from build123d import *

# Parameters (mm, degrees)
SKETCH1_W           = 140.208
SKETCH1_H           = 150
BOSS_EXTRUDE1_DEPTH = 85.725
SKETCH2_W           = 30.48
SKETCH2_H           = 23.9522
SKETCH2_W_2         = 24.384
SKETCH2_H_2         = 17.8562
BOSS_EXTRUDE2_DEPTH = 3.048
SKETCH3_W           = 14.732
SKETCH3_H           = 20.828
BOSS_EXTRUDE3_DEPTH = 5.08
SKETCH4_R           = 1.27
CUT_EXTRUDE1_DEPTH  = 3.81
BOSS_EXTRUDE4_DEPTH = 3.048
SKETCH6_R           = 10.795
BOSS_EXTRUDE5_DEPTH = 25.4
SKETCH7_W           = 24.384
SKETCH7_H           = 17.8562
BOSS_EXTRUDE6_DEPTH = 43.18
SKETCH8_W           = 15.24
SKETCH8_H           = 11.43
BOSS_EXTRUDE7_DEPTH = 17.78
BOSS_EXTRUDE7_TAPER = 5


with BuildPart() as part:
    # Sketch1 → Boss-Extrude1 (new body)
    with BuildSketch(Plane(origin=(0, 0, 0), x_dir=(1, 0, 0), z_dir=(0, 1, 0))):
        with Locations((-120.400582929, 25.928824242)):
            Rectangle(SKETCH1_W, SKETCH1_H)
    extrude(amount=BOSS_EXTRUDE1_DEPTH)

    # Sketch2 → Boss-Extrude2 (add)
    with BuildSketch(Plane(origin=(-50.296582929, 0, 0), x_dir=(0, 0, -1), z_dir=(1, 0, 0))):
        with Locations((-28.243175758, 42.9641)):
            Rectangle(SKETCH2_W, SKETCH2_H)
        with Locations((-28.243175758, 42.9641)):
            Rectangle(SKETCH2_W_2, SKETCH2_H_2, mode=Mode.SUBTRACT)
    extrude(amount=BOSS_EXTRUDE2_DEPTH)

    # Sketch3 → Boss-Extrude3 (add)
    with BuildSketch(Plane(origin=(-50.296582929, 0, 0), x_dir=(0, 0, -1), z_dir=(1, 0, 0))):
        with Locations((-3.097175758, 43.0022)):
            Rectangle(SKETCH3_W, SKETCH3_H)
    extrude(amount=BOSS_EXTRUDE3_DEPTH)

    # Sketch4 → Cut-Extrude1 (cut)
    with BuildSketch(Plane(origin=(-50.296582929, 0, 0), x_dir=(0, 0, -1), z_dir=(1, 0, 0))):
        with Locations((-43.071175758, 6.35)):
            Circle(SKETCH4_R)
        with Locations((94.928824242, 6.35)):
            Circle(SKETCH4_R)
        with Locations((94.928824242, 70.35)):
            Circle(SKETCH4_R)
        with Locations((-19.071175758, 79.725)):
            Circle(SKETCH4_R)
    extrude(amount=-CUT_EXTRUDE1_DEPTH, mode=Mode.SUBTRACT)

    # Sketch5 → Boss-Extrude4 (add)
    with BuildSketch(Plane.ZY.offset(190.504582929)):
        with BuildLine():
            Line((49.071175758, 17.78), (26.211175758, 17.78))
            ThreePointArc((26.211175758, 17.78), (12.622175758, 31.369), (26.211175758, 44.958))
            Line((26.211175758, 44.958), (49.071175758, 44.958))
            Line((49.071175758, 44.958), (49.071175758, 17.78))
        make_face()
    extrude(amount=BOSS_EXTRUDE4_DEPTH)

    # Sketch6 → Boss-Extrude5 (add)
    with BuildSketch(Plane.ZY.offset(193.552582929)):
        with Locations((36.622716845, 31.369)):
            Circle(SKETCH6_R)
    extrude(amount=BOSS_EXTRUDE5_DEPTH)

    # Sketch7 → Boss-Extrude6 (add)
    with BuildSketch(Plane(origin=(-50.296582929, 0, 0), x_dir=(0, 0, -1), z_dir=(1, 0, 0))):
        with Locations((-28.243175758, 42.9641)):
            Rectangle(SKETCH7_W, SKETCH7_H)
    extrude(amount=BOSS_EXTRUDE6_DEPTH)

    # Sketch8 → Boss-Extrude7 (add)
    with BuildSketch(Plane(origin=(-7.116582929, 0, 0), x_dir=(0, 0, -1), z_dir=(1, 0, 0))):
        with Locations((-28.243175758, 42.9641)):
            Rectangle(SKETCH8_W, SKETCH8_H)
    extrude(amount=BOSS_EXTRUDE7_DEPTH, taper=BOSS_EXTRUDE7_TAPER)


solid = part.part
Verification items for the finished model (mm, model axes). A direction names the side the tool comes from. Round coordinates to 2 decimals unless told otherwise and drop trailing zeros. Write each loop counter-clockwise with the first axis right and the second up, starting at its lowest first coordinate (ties: lowest second). Pieces come first, ordered by that corner, then holes.
(1) Section check A-A (z = -43). Enter the section's corners in (x, y) (3 decimals).
Returned:
outline: (-190.505, 0) - (-50.297, 0) - (-50.297, 85.725) - (-190.505, 85.725) - close
(2) Depth check by flat-ended pin: pin 1 Ø3.5 at (x, z) = (-48.5, 26) entering from +Y; pin 2 Ø2 at (y, z) = (63.5, -33) entering from -X; pin 3 Ø19.5 at (x, y) = (-27.5, 41.5) entering from +Z. Enter the tip coordinate at first touch or a pass-through.
Returned:
pin 1: stops at y = 54.94
pin 2: stops at x = -190.5
pin 3: stops at z = 40.44
(3) Mould release check, pull along Z, two halves, no side actions. Record for faces 1 (the flat face through (-47.249, 32, 28)), 2 (the cylindrical face through (-192.007, 31.07, 12.625)), 3 (the flat face through (-121, 0, -27)), 4 (the cylindrical face through (-206.07, 34.61, 46.92)): pulls with the +Z half, pulls with the -Z half, needs draft (parallel to the pull), parting line crosses it, or undercut.
Returned:
face 1: undercut
face 2: pulls with the -Z half
face 3: needs draft
face 4: parting line crosses it
(4) Material ranges on line 1 (Z direction, x = -52, y = 6); line 2 (Z direction, x = -51.35, y = 70.35); line 3 (Z direction, x = -51, y = 70), recorded low to high.
Returned:
line 1: z = -100.93 to -96.15, -93.71 to 41.85, 44.29 to 49.07
line 2: z = -100.93 to -96.2, -93.66 to 49.07
line 3: z = -100.93 to -96.15, -93.71 to 49.07
(5) Access from +Z, -Z, +X, -X, +Y, -Y to the whole of each face (thin tool, end or side, straight path). Record for faces 5 (the flat face through (-7.117, 37, 28)), 6 (the flat face through (-193.553, 38, 27)), 7 (the flat face through (-45.217, 43, 3)), 8 (the flat face through (-48, 53.416, 3)).
Returned:
face 5: +X
face 6: -X
face 7: -Z, +X, +Y, -Y
face 8: -Z, +X, +Y
